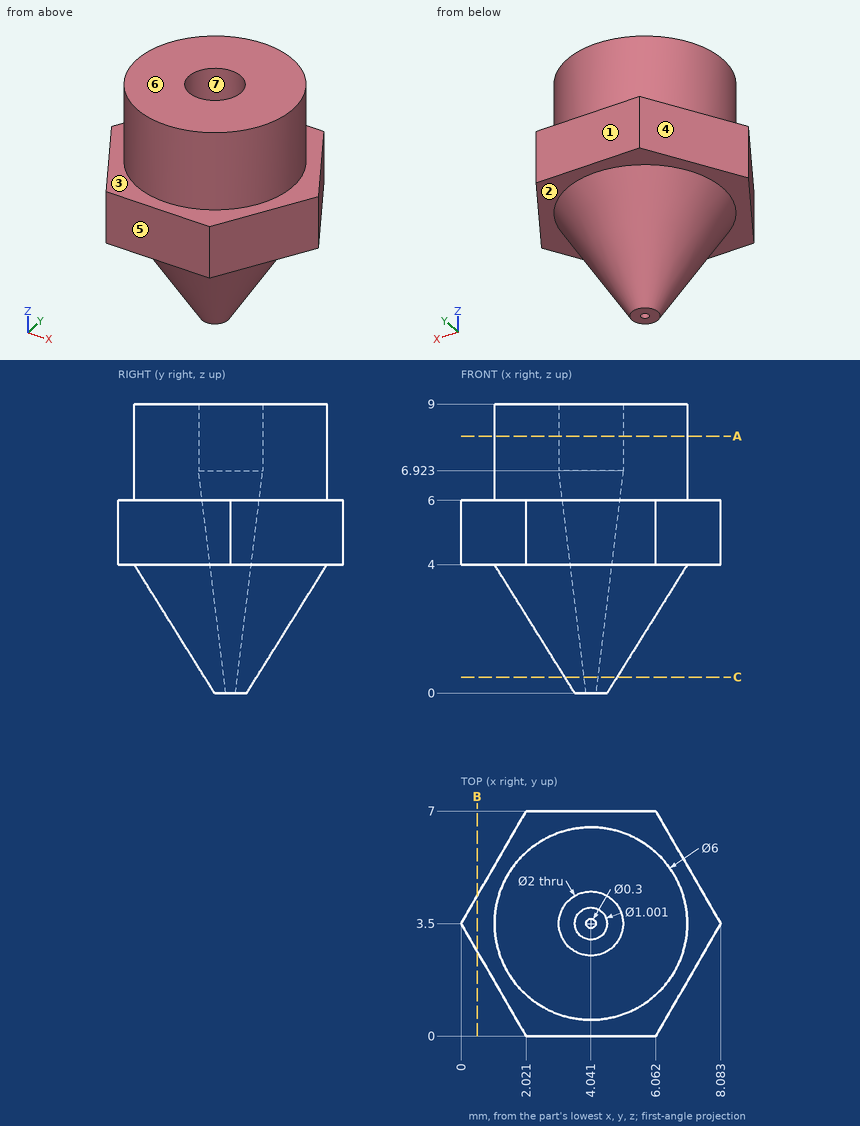
Drawing for the job (mm, zero at the part's lowest x, y, z). A direction names the side the tool comes from. Give positions to 0.01 mm unless a question says otherwise; leave off trailing zeros. Order: outer loops, then holes, each group sorted by start corner. A loop starts at its lowest first (then second) coordinate and runs counter-clockwise, first axis right, second up. Notation, with made-up numbers: (12, 81.5) -> (34, 81.5) arc R25 cw to (34, 108.5) -> close; hole circle Ø3 at (23, 18.25). An arc over 180 degrees is marked (long way). Use one line per item in the form item = value.
(1) Saw through at B-B (x = 0.5). Write the cut outline in (y, z).
Solution:
outline = (2.63, 4) -> (4.37, 4) -> (4.37, 6) -> (2.63, 6) -> close
(2) Saw through at A-A (z = 8). Write the cut outline in (x, y).
Solution:
outline = circle Ø6 at (4.04, 3.5); hole circle Ø2 at (4.04, 3.5)
(3) Pull direction Y, two halves, no side cores. Call the marked faces 4, 5, 6 and 7: +Y half, -Y half, draft (parallel to the pull), parting line (faces both ways), or undercut.
Solution:
face_4 = +Y half
face_5 = -Y half
face_6 = draft
face_7 = undercut
(4) Tool access for the marked faces 1, 2 and 3: list every direction of +Z, -Z, +X, -X, +Y, -Y with a clear straight run to the whole face (end or side of a thin tool).
Solution:
face_1 = +Z, -Z, +X, -X, +Y
face_2 = -Z
face_3 = +Z
(5) Drill centre lines: line 1 (Z direction, x = 7, y = 5.25); line 2 (X direction, y = 4, z = 7) (1 decimal); line 3 (Y direction, x = 4, z = 3.5). Where is each one in solid material? Low to high. Write a range as from..to.
Solution:
line_1 = 4..6
line_2 = 1.1..3.2, 4.9..7
line_3 = 0.81..2.92, 4.08..6.19
(6) Saw through at C-C (z = 0.5). Write the cut outline in (x, y) (1 decimal).
Solution:
outline = circle Ø1.6 at (4, 3.5); hole circle Ø0.4 at (4, 3.5)
